Source: CAD feature listing. Evaluate the final solid. Frame: model axes, mm. Give positions to 0.01 mm unless a question says otherwise; leave off trailing zeros. Order: outer loops, then holes, each group sorted by start corner. A loop starts at its lowest first (then second) coordinate and runs counter-clockwise, first axis right, second up. Notation, with made-up numbers: M 80.5,-8 L 136.5,-8 A25 cw 136.5,7 Z; hole C -15,37 d8. An arc over 180 degrees is marked long. Answer as a JSON object with one key per item and string values. Group by question number.
1. Section query A-A (z = 1.8). Output: boundary loops of the cut face in (x, y), plus the area to 3 significant figures.
2. Section query B-B (x = 8.5). Output: boundary loops of the cut face in (y, z), plus the area to 3 significant figures.
3. Pin query (flat end, axial travel): P1, Ø1, axis at y = -36, z = 0.5, coming from the -X side; P2, Ø1.8, axis at x = -7.87, y = -38.35, coming from the -Z side. Return the tip coordinate at first contact, or that it passes through.
4. Pull-direction query (Y, two-part tool) for faces 1 (the cylindrical face through (-7.06, -37.09, 1.38)), 2 (the flat face through (-9, -10, 0)), 3 (the flat face through (-32.4, -0.6, 1.4)), 4 (the flat face through (-21.8, -21.85, 1.38)); classes: +Y half, -Y half, draft (parallel to the pull), parting line (faces both ways), or undercut.
5. Section query C-C (y = -6). Output: boundary loops of the cut face in (x, z).
6. Material intervals for L1, parallel to X at y = -3.5, z = 2.2; L2, parallel to Z at x = -29, y = -4; L3, parallel to Y at x = -6, z = 1.95, sorted ascending. Write a range as [from, to].
from build123d import *

# Parameters (mm, degrees)
F0_R     = 1.5
F0_R_2   = 6.5
F1_DEPTH = 3
F2_SIZE  = 0.2


with BuildPart() as f1:
    # F0 (on Top) → F1 (new body)
    with BuildSketch(Plane.XY):
        Polygon((-5.761886, -41.850388), (15.147641, -2.238909), (13.106366, 1.146824), (-31.408452, 1.146824), (-33.420278, -2.398261), (-9.855032, -41.850388), align=None)
        with Locations((-7.870373, -38.353176)):
            Circle(F0_R, mode=Mode.SUBTRACT)
        with Locations((-6.920373, -20.853176)):
            Circle(F0_R_2, mode=Mode.SUBTRACT)
        with Locations((-29.370373, -2.353176)):
            Circle(F0_R, mode=Mode.SUBTRACT)
        with Locations((11.129627, -2.353176)):
            Circle(F0_R, mode=Mode.SUBTRACT)
    extrude(amount=F1_DEPTH)

    # F2
    f2_edges = [f1.edges().sort_by_distance(p)[0] for p in [
        (-21.637655, -22.124324, 3),
        (-7.808459, -41.850388, 3),
        (4.692878, -22.044649, 3),
        (14.127004, -0.546043, 3),
        (-9.151043, 1.146824, 3),
        (-32.414365, -0.625718, 3),
        (-9.370373, -38.353176, 3),
        (-13.420373, -20.853176, 3),
        (-30.870373, -2.353176, 3),
        (9.629627, -2.353176, 3),
    ]]
    chamfer(f2_edges, length=F2_SIZE)


solid = f1.part
Answer sheet:
{
 "1": {"outline": "M -33.42,-2.4 L -9.86,-41.85 L -5.76,-41.85 L 15.15,-2.24 L 13.11,1.15 L -31.41,1.15 Z; hole C -29.37,-2.35 d3; hole C -6.92,-20.85 d13; hole C -7.87,-38.35 d3; hole C 11.13,-2.35 d3", "area": "1,050 mm^2"},
 "2": {"outline": "M -14.83,0 L 1.15,0 L 1.15,2.8 L 0.95,3 L -14.4,3 L -14.83,2.8 Z", "area": "47.9 mm^2"},
 "3": {"P1": "x = -13.65", "P2": "through"},
 "4": {"face 1": "undercut", "face 2": "draft", "face 3": "+Y half", "face 4": "-Y half"},
 "5": {"outline": "M -31.27,0 L 13.16,0 L 13.16,2.8 L 12.94,3 L -31.04,3 L -31.27,2.8 Z"},
 "6": {"L1": "[-32.76, -30.34], [-28.4, 10.16], [12.1, 14.48]", "L2": "[0, 2.99]", "L3": "[-41.85, -27.29], [-14.42, 1.15]"}
}
